Part print with two shaded views. Sizes in mm from the minimum x, y, z corner. A direction names the side the tool comes from. Give positions to 0.01 mm unless a question says otherwise; leave off trailing zeros. Loops run counter-clockwise (first coordinate to the right, second up) from the corner with the lowest first, then second, coordinate; pieces in that order, holes last. Notation, with made-up numbers: M -6,-33 L 50,-33 A22 ccw 50,-1 Z; hole C 1,-3.5 d6. An arc over 180 degrees is marked long. Answer as a JSON object with one key per item and string values. Group by question number.
1. Slice it at D-D (x = 165.5). List the corners of the cut face in (y, z), then the cut area to 3 significant figures.
2. Mould opens along Y. For the marked faces 5, 6 and 7 say: released by +Y, released by -Y, zero draft, split by the parting line, or undercut.
3. Drill centre lines: line 1 along Y through (x, z) = (128, 450); line 2 along Y through (x, z) = (113, 129); line 3 along Z through (x, y) = (173, 279). Where is each one in solid material? Low to high. Write a range as [from, to].
4. Slice it at B-B (x = 138.5). List the corners of the cut face in (y, z).
5. Slice it at A-A (y = 150). List the corners of the cut face in (x, z).
6. 3-axis set-ups, long thin cutter, end or side, ignore diameter. For the marked faces 1, 2, 3 and 4: which of +Z, -Z, +X, -X, +Y, -Y reach the whole face in a straight line?
7. Drop flat-ended pins along their axis: pin 1 Ø22.5 at (y, z) = (262.5, 51.5) entering from +X; pin 2 Ø15 at (x, y) = (25.5, 30.5) entering from -Z; pin 3 Ø5 at (x, y) = (158, 135.5) entering from +Z; pin 4 Ø8 at (y, z) = (188, 424.5) entering from -X (3 decimals). Give the stop position or say it passes through.
8. Slice it at C-C (z = 493.5). List the corners of the cut face in (x, y).
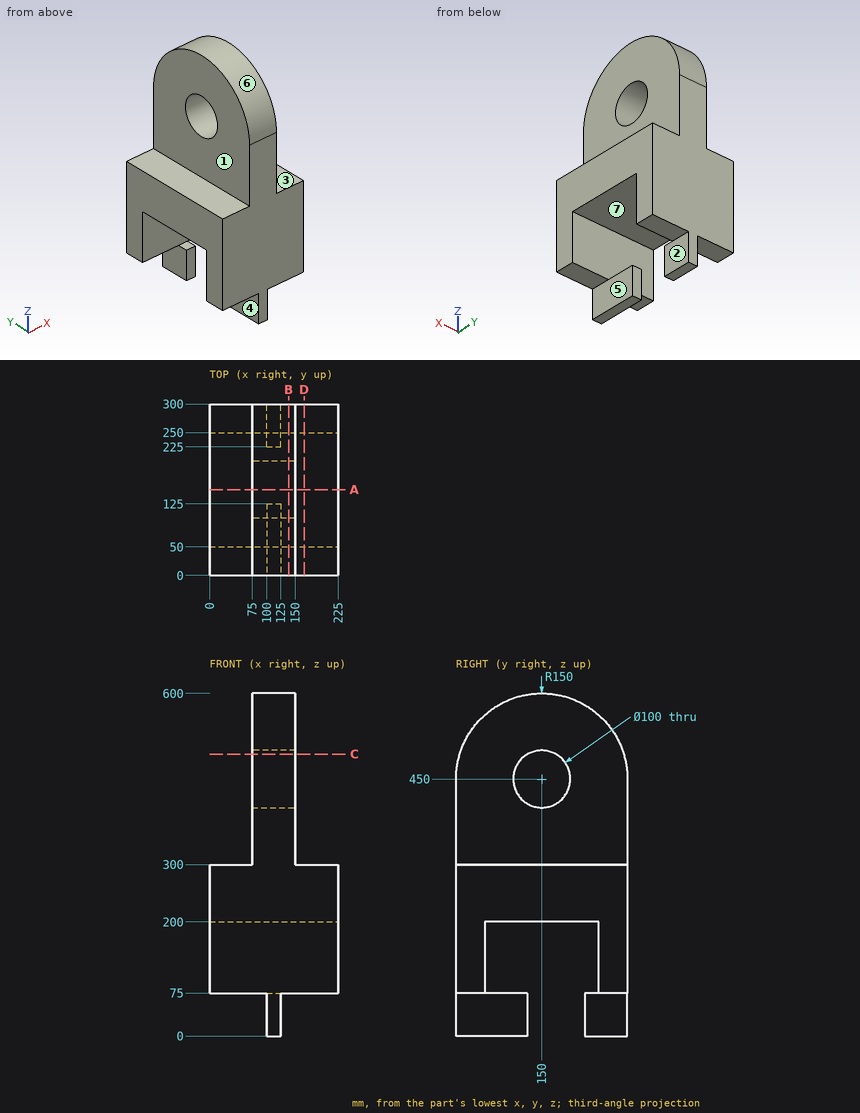
Established:
{
 "1": {"outline": "M 0,75 L 50,75 L 50,200 L 250,200 L 250,75 L 300,75 L 300,300 L 0,300 Z", "area": "42,500 mm^2"},
 "2": {"face 5": "zero draft", "face 6": "split by the parting line", "face 7": "undercut"},
 "3": {"line 1": "y = [0, 100], [200, 300]", "line 2": "y = [0, 50], [250, 300]", "line 3": "z = [75, 300]"},
 "4": {"outline": "M 0,75 L 50,75 L 50,200 L 250,200 L 250,75 L 300,75 L 300,450 A150 ccw 0,450 Z; hole C 150,450 d100"},
 "5": {"outline": "M 0,200 L 225,200 L 225,300 L 150,300 L 150,400 L 75,400 L 75,300 L 0,300 Z; M 75,500 L 150,500 L 150,600 L 75,600 Z"},
 "6": {"face 1": "+Z, -X, +Y, -Y", "face 2": "-Z, +X, +Y, -Y", "face 3": "+Z, +X, +Y, -Y", "face 4": "-Z, -X, +Y, -Y"},
 "7": {"pin 1": "stops at x = 125", "pin 2": "stops at z = 75", "pin 3": "stops at z = 300", "pin 4": "passes through"},
 "8": {"outline": "M 75,6.45 L 150,6.45 L 150,125.35 L 75,125.35 Z; M 75,174.65 L 150,174.65 L 150,293.55 L 75,293.55 Z"}
}
